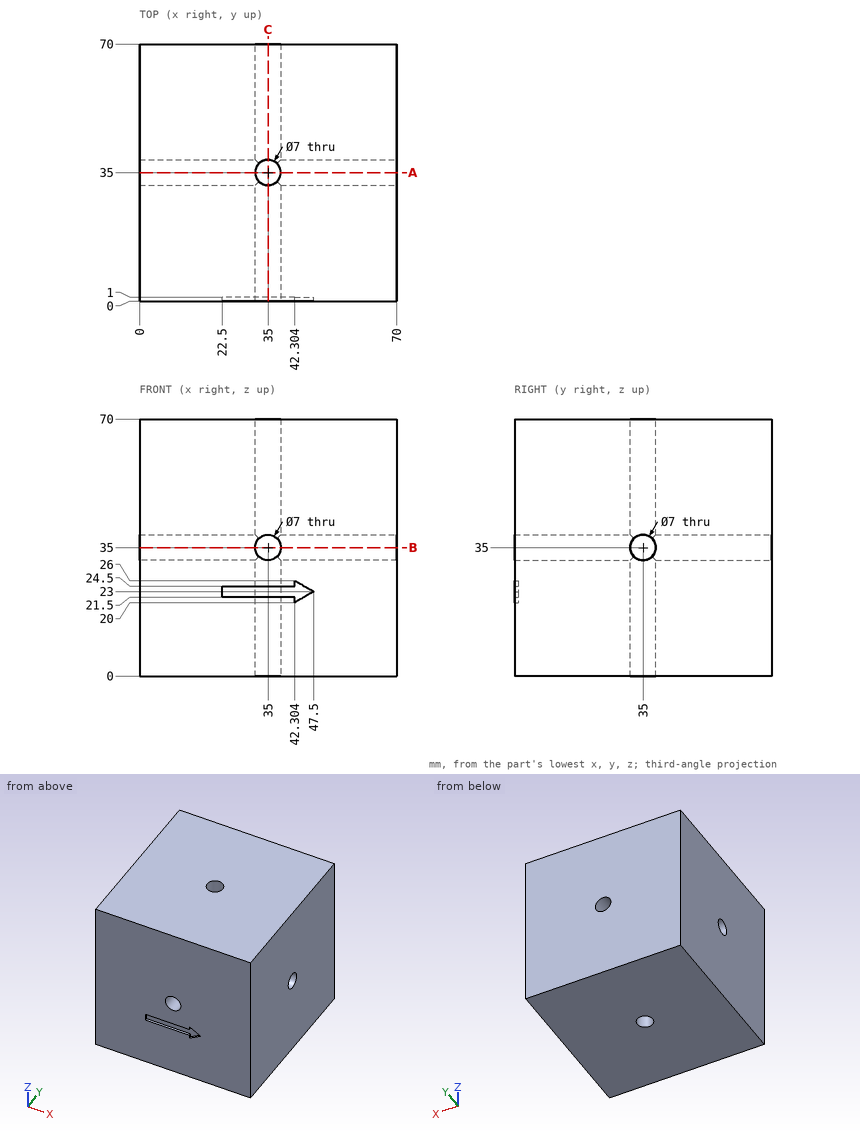
Here's the drawing with two shaded views (mm, measured from the low corner). I have some questions. Coordinates: 2 decimals unless noted, no trailing zeros. Order: outer loops, then holes, each group sorted by start corner. A loop starts at its lowest first (then second) coordinate and runs counter-clockwise, first axis right, second up. Notation, with made-up numbers: (69, -32.75) - (88, -32.75) arc R14 ccw to (88, -19.75) - close; hole circle Ø10 at (-31, 4.5). An arc over 180 degrees is marked (long way). Answer in a Markdown table with one row per item.
1. Suppose I cut it at A-A (y = 35). Please give me the cut outline in (x, z), and give its area (3 significant figures).
Reply:
| item | result |
|---|---|
| outline | (0, 0) - (31.5, 0) - (31.5, 31.5) - (0, 31.5) - close; (0, 38.5) - (31.5, 38.5) - (31.5, 70) - (0, 70) - close; (38.5, 0) - (70, 0) - (70, 31.5) - (38.5, 31.5) - close; (38.5, 38.5) - (70, 38.5) - (70, 70) - (38.5, 70) - close |
| area | 3,970 mm^2 |
2. If I drill on line 1 along Z through (x, y) = (35, 22.5), over which ranges is the centre line in solid material (lowest first)?
Reply:
| item | result |
|---|---|
| line 1 | z = 0 to 31.5, 38.5 to 70 |
3. Suppose I cut it at C-C (x = 35). Please give me the cut outline in (y, z).
Reply:
| item | result |
|---|---|
| outline | (0, 0) - (31.5, 0) - (31.5, 31.5) - (0, 31.5) - (0, 24.5) - (1, 24.5) - (1, 21.5) - (0, 21.5) - close; (0, 38.5) - (31.5, 38.5) - (31.5, 70) - (0, 70) - close; (38.5, 0) - (70, 0) - (70, 31.5) - (38.5, 31.5) - close; (38.5, 38.5) - (70, 38.5) - (70, 70) - (38.5, 70) - close |
